Part model, mm, in its own coordinate system. A direction names the side the tool comes from. Round coordinates to 2 decimals unless told otherwise and drop trailing zeros. Loops run counter-clockwise (first coordinate to the right, second up) from the corner with the lowest first, then second, coordinate; pieces in that order, holes last.
from build123d import *

# Parameters (mm, degrees)
F0_R     = 1.5875
F1_DEPTH = 3.048


with BuildPart() as f1:
    # F0 (on Right) → F1 (new body)
    with BuildSketch(Plane.YZ):
        with BuildLine():
            ThreePointArc((20.6192658602, 94.538977478), (23.3833367864, 87.7571874382), (30.1439925328, 84.9418192372))
            ThreePointArc((30.1439925328, 84.9418192372), (36.8791846236, 87.7316271464), (39.6689925328, 94.4668192372))
            ThreePointArc((39.6689925328, 94.4668192372), (39.6560750954, 94.9627126954), (39.6173578196, 95.4572611305))
            Line((39.6173578196, 95.4572611305), (39.5927784781, 95.6693453948))
            ThreePointArc((39.5927784781, 95.6693453948), (29.577534542, 103.9749605038), (20.6192658602, 94.538977478))
        make_face()
        with BuildLine():
            ThreePointArc((33.3189925328, 94.4668192372), (32.3890565631, 92.221755207), (30.1439925328, 91.2918192372))
            ThreePointArc((30.1439925328, 91.2918192372), (27.8989285025, 96.7118832675), (33.3189925328, 94.4668192372))
        make_face(mode=Mode.SUBTRACT)
        with BuildLine():
            ThreePointArc((39.6689925328, 94.4668192372), (36.8791846236, 87.7316271464), (30.1439925328, 84.9418192372))
            Line((30.1439925328, 84.9418192372), (30.1439925328, 59.5418192372))
            ThreePointArc((30.1439925328, 59.5418192372), (39.1285508172, 56.754727299), (44.9583639095, 49.3720822211))
            Line((44.9583639095, 49.3720822211), (39.6173578196, 95.4572611305))
            ThreePointArc((39.6173578196, 95.4572611305), (39.6560750954, 94.9627126954), (39.6689925328, 94.4668192372))
        make_face()
        with Locations((35.2487452328, 80.1920192372)):
            Circle(F0_R, mode=Mode.SUBTRACT)
        with BuildLine():
            Line((30.1439925328, 59.5418192372), (30.1439925328, 84.9418192372))
            ThreePointArc((30.1439925328, 84.9418192372), (23.3833367864, 87.7571874382), (20.6192658602, 94.538977478))
            Line((20.6192658602, 94.538977478), (15.9762797521, 50.8286304302))
            ThreePointArc((15.9762797521, 50.8286304302), (21.8276870937, 57.1891965742), (30.1439925328, 59.5418192372))
        make_face()
        with BuildLine():
            ThreePointArc((44.9583639095, 49.3720822211), (39.1285508172, 56.754727299), (30.1439925328, 59.5418192372))
            Line((30.1439925328, 59.5418192372), (30.1439925328, 46.8418192372))
            ThreePointArc((30.1439925328, 46.8418192372), (32.3890565631, 45.9118832675), (33.3189925328, 43.6668192372))
            ThreePointArc((33.3189925328, 43.6668192372), (32.3890565631, 41.421755207), (30.1439925328, 40.4918192372))
            Line((30.1439925328, 40.4918192372), (30.1439925328, 27.7918192372))
            ThreePointArc((30.1439925328, 27.7918192372), (40.2348384207, 31.4115977269), (45.7239045432, 40.6201872035))
            Line((45.7239045432, 40.6201872035), (46.0162507225, 43.3717854106))
            ThreePointArc((46.0162507225, 43.3717854106), (46.0183070654, 43.519295954), (46.0189925328, 43.6668192372))
            ThreePointArc((46.0189925328, 43.6668192372), (45.7515831637, 46.5683256904), (44.9583639095, 49.3720822211))
        make_face()
        with BuildLine():
            Line((30.1439925328, 46.8418192372), (30.1439925328, 59.5418192372))
            ThreePointArc((30.1439925328, 59.5418192372), (21.8276870937, 57.1891965742), (15.9762797521, 50.8286304302))
            ThreePointArc((15.9762797521, 50.8286304302), (14.5245790346, 46.5039915923), (14.362635633, 41.9450761088))
            Line((14.362635633, 41.9450761088), (14.4599248422, 41.2121001744))
            ThreePointArc((14.4599248422, 41.2121001744), (19.8229712685, 31.6048067575), (30.1439925328, 27.7918192372))
            Line((30.1439925328, 27.7918192372), (30.1439925328, 40.4918192372))
            ThreePointArc((30.1439925328, 40.4918192372), (26.9689925328, 43.6668192372), (30.1439925328, 46.8418192372))
        make_face()
        with BuildLine():
            ThreePointArc((39.6173578196, 95.4572611305), (39.6056624037, 95.5633721334), (39.5927784781, 95.6693453948))
            Line((39.5927784781, 95.6693453948), (39.6173578196, 95.4572611305))
        make_face()
        with BuildLine():
            Line((14.4599248422, 41.2121001744), (14.362635633, 41.9450761088))
            ThreePointArc((14.362635633, 41.9450761088), (14.4070122128, 41.578021639), (14.4599248422, 41.2121001744))
        make_face()
        with BuildLine():
            ThreePointArc((45.7239045432, 40.6201872035), (40.2348384207, 31.4115977269), (30.1439925328, 27.7918192372))
            Line((30.1439925328, 27.7918192372), (30.1439925328, -10.3081807628))
            ThreePointArc((30.1439925328, -10.3081807628), (36.2027481756, -12.4835477746), (39.4940461474, -18.0160064718))
            Line((39.4940461474, -18.0160064718), (45.7239045432, 40.6201872035))
        make_face()
        with BuildLine():
            Line((30.1439925328, -10.3081807628), (30.1439925328, 27.7918192372))
            ThreePointArc((30.1439925328, 27.7918192372), (19.8229712685, 31.6048067575), (14.4599248422, 41.2121001744))
            Line((14.4599248422, 41.2121001744), (20.2870354782, -2.6892933731))
            ThreePointArc((20.2870354782, -2.6892933731), (18.4004499897, -8.9575963205), (12.4498462988, -11.6854420564))
            Line((12.4498462988, -11.6854420564), (-13.5119950672, -11.8287714378))
            ThreePointArc((-13.5119950672, -11.8287714378), (-8.4193114637, -14.4019187635), (-6.3685074672, -19.7264578433))
            ThreePointArc((-6.3685074672, -19.7264578433), (-6.3685131868, -19.7359866548), (-6.3685303455, -19.7455154525))
            Line((-6.3685303455, -19.7455154525), (20.6190199868, -19.8103116316))
            ThreePointArc((20.6190199868, -19.8103116316), (23.4168907599, -13.0899080605), (30.1439925328, -10.3081807628))
        make_face()
        with BuildLine():
            ThreePointArc((45.7239045432, 40.6201872035), (45.9301439241, 41.9896045066), (46.0162507225, 43.3717854106))
            Line((46.0162507225, 43.3717854106), (45.7239045432, 40.6201872035))
        make_face()
        with BuildLine():
            ThreePointArc((39.4940461474, -18.0160064718), (36.2027481756, -12.4835477746), (30.1439925328, -10.3081807628))
            Line((30.1439925328, -10.3081807628), (30.1439925328, -16.6581807628))
            ThreePointArc((30.1439925328, -16.6581807628), (32.3890565631, -17.5881167325), (33.3189925328, -19.8331807628))
            ThreePointArc((33.3189925328, -19.8331807628), (30.1401810082, -23.0081784749), (26.9690016841, -19.8255577191))
            Line((26.9690016841, -19.8255577191), (20.6190199868, -19.8103116316))
            ThreePointArc((20.6190199868, -19.8103116316), (21.6276394845, -24.0990166429), (24.4582910855, -27.4750669208))
            ThreePointArc((24.4582910855, -27.4750669208), (34.4200490522, -28.3444066229), (39.6689925328, -19.8331807628))
            ThreePointArc((39.6689925328, -19.8331807628), (39.6251550586, -18.9203926382), (39.4940461474, -18.0160064718))
        make_face()
        with BuildLine():
            ThreePointArc((24.4582910855, -27.4750669208), (21.6276394845, -24.0990166429), (20.6190199868, -19.8103116316))
            Line((20.6190199868, -19.8103116316), (-6.3685303455, -19.7455154525))
            ThreePointArc((-6.3685303455, -19.7455154525), (-8.1205720343, -24.7008215972), (-12.5846813465, -27.4750669208))
            Line((-12.5846813465, -27.4750669208), (24.4582910855, -27.4750669208))
        make_face()
        with BuildLine():
            ThreePointArc((-12.5846813465, -27.4750669208), (-8.1205720343, -24.7008215972), (-6.3685303455, -19.7455154525))
            ThreePointArc((-6.3685303455, -19.7455154525), (-6.3685131868, -19.7359866548), (-6.3685074672, -19.7264578433))
            ThreePointArc((-6.3685074672, -19.7264578433), (-8.4193114637, -14.4019187635), (-13.5119950672, -11.8287714378))
            ThreePointArc((-13.5119950672, -11.8287714378), (-22.229603403, -20.1960679971), (-12.5846813465, -27.4750669208))
        make_face()
        with BuildLine():
            ThreePointArc((-11.1310074672, -19.7264578433), (-11.131009755, -19.7302693679), (-11.1310166185, -19.734080887))
            ThreePointArc((-11.1310166185, -19.734080887), (-17.4810051794, -19.7226463187), (-11.1310074672, -19.7264578433))
        make_face(mode=Mode.SUBTRACT)
        with BuildLine():
            Line((30.1439925328, -16.6581807628), (30.1439925328, -10.3081807628))
            ThreePointArc((30.1439925328, -10.3081807628), (23.4168907599, -13.0899080605), (20.6190199868, -19.8103116316))
            Line((20.6190199868, -19.8103116316), (26.9690016841, -19.8255577191))
            ThreePointArc((26.9690016841, -19.8255577191), (27.9016252752, -17.5854231953), (30.1439925328, -16.6581807628))
        make_face()
    extrude(amount=-F1_DEPTH)


solid = f1.part
1) Slice it at B-B, the plane z = -8. Give the cut face in (x, y), then the cut area to 3 significant figures.
Values:
outline: (-3.05, 19.12) - (0, 19.12) - (0, 40.56) - (-3.05, 40.56) - close
area: 65.4 mm2
2) Drop flat-ended pins along their axis: pin 1 Ø1.5 at (x, z) = (-0.5, 64.5) entering from -Y; pin 2 Ø1.5 at (x, y) = (-1, 2) entering from -Z. Give the stop position or say it passes through.
Values:
pin 1: stops at y = 17.35
pin 2: stops at z = -27.48
3) Tool access for faces 1 (the face through (-1.5, 18.33, 72.99)), 2 (the face through (-1.5, 18.46, -8.89)), 3 (the face through (-2, 6, -27.475)): list every direction of +Z, -Z, +X, -X, +Y, -Y with a clear straight run to the whole face (end or side of a thin tool).
Values:
face 1: +Z, +X, -X, -Y
face 2: +X, -X, -Y
face 3: -Z, +X, -X
4) Slice it at C-C, the plane y = -5.5. Give the cut face in (x, z), then the cut area to 3 significant figures.
Values:
outline: (-3.05, -27.48) - (0, -27.48) - (0, -11.78) - (-3.05, -11.78) - close
area: 47.8 mm2
5) Mould opens along Y. For faces 4 (the face through (0, 27, 23)), 5 (the face through (-1.5, -17.48, -19.86)), 6 (the face through (-1.503, 42.325, 72.092)) say: released by +Y, released by -Y, zero draft, split by the parting line, or undercut.
Values:
face 4: zero draft
face 5: undercut
face 6: released by +Y
6) Slice it at A-A, the plane x = -0.5. Give the number of separate pieces and of enclosed holes in the cut face, then the cut area to 3 significant figures.
Values:
separate pieces: 1
enclosed holes: 5
area: 3,650 mm2
7) Wall check: line 1 along Z through (x, y) = (-1.6, 30); line 2 along Y through (x, z) = (-1.95, -22.5); line 3 along Y through (x, z) = (-0.3, 92). Give the ranges that are in metal, low to high.
Values:
line 1: z = -29.36 to -23, -16.66 to 40.5, 46.84 to 91.3, 97.64 to 103.99
line 2: y = -21.74 to -15.85, -12.76 to 28.42, 31.87 to 39.29
line 3: y = 20.35 to 28.15, 32.14 to 40.02
